Verification items for the finished model (mm, model axes). Coordinates: 2 decimals unless noted, no trailing zeros. Order: outer loops, then holes, each group sorted by start corner. A loop starts at its lowest first (then second) coordinate and runs counter-clockwise, first axis right, second up. Notation, with made-up numbers: M 78.5,69.25 L 84.5,69.25 A22 cw 84.5,96.25 Z; hole C -30.5,4.25 d11. An arc over 180 degrees is marked long. Return JSON: item names as keys, results as strings.
```python
from build123d import *

# Parameters (mm, degrees)
SKETCH1_W                                         = 80
SKETCH1_H                                         = 20
BOSS_EXTRUDE1_DEPTH                               = 20
SKETCH2_R                                         = 7.5
CUT_EXTRUDE1_DEPTH                                = 20
CSK_FOR_8_FLAT_HEAD_MACHINE_SCREW_100_D           = 4.4958
CSK_FOR_8_FLAT_HEAD_MACHINE_SCREW_100_CSINK_D     = 8.4328
CSK_FOR_8_FLAT_HEAD_MACHINE_SCREW_100_CSINK_ANGLE = 100


with BuildPart() as part:
    # Sketch1 → Boss-Extrude1 (new body)
    with BuildSketch(Plane(origin=(0, 0, 0), x_dir=(1, 0, 0), z_dir=(0, 1, 0))):
        Rectangle(SKETCH1_W, SKETCH1_H)
    extrude(amount=BOSS_EXTRUDE1_DEPTH)

    # Sketch2 → Cut-Extrude1 (cut)
    with BuildSketch(Plane.XY.offset(10)):
        with Locations((-5, 10)):
            Circle(SKETCH2_R)
        with Locations((5, 10)):
            Circle(SKETCH2_R)
    extrude(amount=-CUT_EXTRUDE1_DEPTH, mode=Mode.SUBTRACT)

    # CSK for #8 Flat Head Machine Screw (100)1 (through all)
    with Locations(Plane(origin=(0, 20, 0), x_dir=(1, 0, 0), z_dir=(0, 1, 0))):
        with Locations((-30, 0), (30, 0)):
            CounterSinkHole(CSK_FOR_8_FLAT_HEAD_MACHINE_SCREW_100_D / 2, CSK_FOR_8_FLAT_HEAD_MACHINE_SCREW_100_CSINK_D / 2, counter_sink_angle=CSK_FOR_8_FLAT_HEAD_MACHINE_SCREW_100_CSINK_ANGLE)


solid = part.part
```
Q1. Cross-section at C-C, the plane z = 0. Record the boundary of the cut face in (x, y).
Values:
{"outline": "M -40,0 L -32.25,0 L -32.25,18.35 L -34.22,20 L -40,20 Z; M -27.75,0 L 27.75,0 L 27.75,18.35 L 25.78,20 L -25.78,20 L -27.75,18.35 Z; M 32.25,0 L 40,0 L 40,20 L 34.22,20 L 32.25,18.35 Z; hole M 0,4.41 A7.5 ccw long 0,15.59 A7.5 ccw long Z"}
Q2. Material ranges on line 1 along Z through (x, y) = (-30, 4.5); line 2 along X through (y, z) = (11.5, -1.75); line 3 along X through (y, z) = (16.5, 6), recorded low to high.
Values:
{"line 1": "-10 to -2.25, 2.25 to 10", "line 2": "-40 to -31.41, -28.59 to -12.35, 12.35 to 28.59, 31.41 to 40", "line 3": "-40 to -8.74, -1.26 to 1.26, 8.74 to 40"}
Q3. Cross-section at B-B, the plane x = 9.5. Record the boundary of the cut face in (y, z).
Values:
{"outline": "M 0,-10 L 4,-10 L 4,10 L 0,10 Z; M 16,-10 L 20,-10 L 20,10 L 16,10 Z"}
Q4. Cross-section at A-A, the plane y = 10. Record the boundary of the cut face in (x, z), and give its area (3 significant figures).
Values:
{"outline": "M -40,-10 L -12.5,-10 L -12.5,10 L -40,10 Z; M 12.5,-10 L 40,-10 L 40,10 L 12.5,10 Z; hole C -30,0 d4.5; hole C 30,0 d4.5", "area": "1,070 mm^2"}
Q5. Go/stop test with a flat-tipped pin: pin 1 (2 mm diameter, centred on x = -28.5, z = 1, fed in from +Y). Record where the tip stops, or that it passes through.
Values:
{"pin 1": "y = 18.81"}
Q6. Cross-section at D-D, the plane x = 30. Record the boundary of the cut face in (y, z), and give its area (3 significant figures).
Values:
{"outline": "M 0,-10 L 20,-10 L 20,-4.22 L 18.35,-2.25 L 0,-2.25 Z; M 0,2.25 L 18.35,2.25 L 20,4.22 L 20,10 L 0,10 Z", "area": "307 mm^2"}
Q7. Draft check along Y on faces 1 (the face through (12.496, 9.758, 0.14)), 2 (the face through (-12.496, 10.242, 0.14)), 3 (the face through (-1, 20, 0)), 4 (the face through (-40, 10, 0)). Enter one of: pulls with the +Y half, pulls with the -Y half, needs draft (parallel to the pull), parting line crosses it, or undercut.
Values:
{"face 1": "undercut", "face 2": "undercut", "face 3": "pulls with the +Y half", "face 4": "needs draft"}
